Autodesk Inventor part; units mm, degrees
ref_plane "YZ Plane" through (0, 0, 0) normal (1, 0, 0) x (0, 1, 0)
ref_plane "XZ Plane" through (0, 0, 0) normal (0, 1, 0) x (-1, 0, 0)
ref_plane "XY Plane" through (0, 0, 0) normal (0, 0, 1) x (1, 0, 0)
sketch "Sketch1" plane through (0, 0, 0) normal (0, 0, 1) x (1, 0, 0)
  circle A0 centre (202.1451, 12.6471) radius 3.9688
  circle A1 centre (202.1451, -12.7529) radius 3.9688
  circle A2 centre (176.7451, 12.6471) radius 3.9688
  circle A3 centre (176.7451, -12.7529) radius 3.9688
  line L0 (211.6701, 22.1721) -> (167.2201, 22.1721)
  line L1 (167.2201, 22.1721) -> (167.2201, -22.2779)
  line L2 (167.2201, -22.2779) -> (211.6701, -22.2779)
  line L3 (211.6701, -22.2779) -> (211.6701, 22.1721)
  point P0 (0, 0)
  dimension "d0" = 9.525
  dimension "d1" = 9.525
  dimension "d2" = 44.45
  dimension "d3" = 44.45
extrude "Extrusion1" add sketch "Sketch1" along normal blind 38.1
sketch "Sketch2" plane through (0, 0, 38.1) normal (0, 0, 1) x (1, 0, 0)
  line L0 (211.6701, -22.2779) -> (211.6701, 22.1721)
  line L1 (167.2201, 22.1721) -> (167.2201, -22.2779)
  line L2 (211.6701, 22.1721) -> (167.2201, 22.1721)
  line L3 (167.2201, 22.1721) -> (167.2201, -22.2779)
  line L4 (167.2201, -22.2779) -> (211.6701, -22.2779)
  line L5 (211.6701, -22.2779) -> (211.6701, 22.1721)
  point P0 (0, 0)
extrude "Extrusion2" add sketch "Sketch2" along normal blind 165.1
sketch "Sketch3" plane through (167.2201, -22.2779, 0) normal (-1, 0, 0) x (0, 0, 1)
  point P0 (0, 22.2779)
sketch "Sketch4" plane through (211.6701, -22.2779, 0) normal (1, 0, 0) x (0, 0, -1)
  circle A0 centre (-127, 22.2779) radius 17.4625
  point P0 (0, 22.2779)
  dimension "d8" = 34.925
  dimension "d11" = 127
extrude "Extrusion3" cut sketch "Sketch4" against normal blind 7.1437
sketch "Sketch5" plane through (204.5263, 0, 127) normal (1, 0, 0) x (0, 0, -1)
  circle A0 centre (0, 0) radius 9.525
  point P0 (127, 0)
  dimension "d12" = 19.05
extrude "Extrusion4" cut sketch "Sketch5" against normal blind 50.8
sketch "Sketch6" plane through (167.2201, -22.2779, 0) normal (0, -1, 0) x (1, 0, 0)
  circle A0 centre (22.225, 171.45) radius 12.7
  line L0 (0, 203.2) -> (44.45, 203.2)
  point P0 (-167.2201, 0)
  dimension "d15" = 25.4
  dimension "d16" = 31.75
extrude "Extrusion5" cut sketch "Sketch6" against normal blind 50.8
sketch "Sketch7" plane through (167.2201, -22.2779, 0) normal (0, -1, 0) x (1, 0, 0)
  line L0 (44.45, 203.2) -> (0, 203.2)
  line L1 (23.8125, 203.2) -> (20.6375, 203.2)
  line L2 (20.6375, 203.2) -> (20.6375, 177.8)
  line L3 (20.6375, 177.8) -> (23.8125, 177.8)
  line L4 (23.8125, 177.8) -> (23.8125, 203.2)
  line L5 (44.45, 0) -> (44.45, 203.2)
  point P0 (-167.2201, 0)
  dimension "d19" = 3.175
  dimension "d20" = 20.6375
  dimension "d21" = 25.4
extrude "Extrusion6" cut sketch "Sketch7" against normal blind 50.8
sketch "Sketch8" plane through (211.6701, -22.2779, 0) normal (1, 0, 0) x (0, 0, -1)
  circle A0 centre (-193.675, 31.75) radius 6.35
  line L0 (-203.2, 0) -> (-203.2, 44.45)
  circle A1 centre (-193.675, 12.7) radius 6.35
  line L1 (0, 44.45) -> (-203.2, 44.45)
  line L2 (0, 0) -> (-203.2, 0)
  point P0 (0, 22.2779)
  dimension "d24" = 12.7
  dimension "d25" = 9.525
  dimension "d26" = 12.7
  dimension "d27" = 12.7
  dimension "d28" = 12.7
extrude "Extrusion7" cut sketch "Sketch8" against normal blind 7.9375
sketch "Sketch9" plane through (203.7326, 9.4721, 193.675) normal (1, 0, 0) x (0, 0, -1)
  circle A0 centre (0, 0) radius 6.35
  circle A1 centre (0, 0) radius 3.9688
  circle A2 centre (0, -19.05) radius 6.35
  circle A3 centre (0, -19.05) radius 3.9688
  point P0 (193.675, -9.4721)
  dimension "d31" = 7.9375
  dimension "d32" = 7.9375
extrude "Extrusion8" cut sketch "Sketch9" against normal blind 38.1 contours A1 | A3
properties part number "Corner Stand"
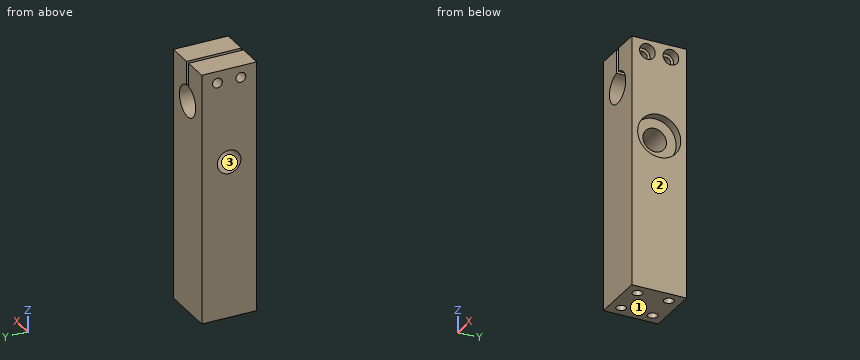
For this review, take the finished solid that the model builds, in its own axes (mm). Face numbers are marked on the shaded views. Coordinates: 2 decimals unless noted, no trailing zeros. Write each loop counter-clockwise with the first axis right and the second up, starting at its lowest first coordinate (ties: lowest second). Pieces come first, ordered by that corner, then holes. Notation, with made-up numbers: (66, 3.5) - (78, 3.5) arc R23 ccw to (78, 30.5) - close; hole circle Ø1 at (88.25, 67.5). An arc over 180 degrees is marked (long way). Answer in a Markdown table with one row per item. Add a question column.
Q1. For probe 1 along Z at (x, y) = (183.5, 6.5); probe 2 along Z at (x, y) = (208, -4); probe 3 along X at (y, z) = (-9.5, 131), list the stretches that pass through material, from the lowest coordinate up.
Q2. We need section D-D, the plane z = 18. State the section outline as (x, y) points, and give its area (3 significant figures).
Q3. Draft analysis for pull direction Z (two halves, no side actions). For the marked faces 1, 2 and 3, state which applies: +Z half, -Z half, draft (parallel to the pull), parting line (faces both ways), or undercut.
Q4. For P1, Ø6.5, axis at y = 9.47, z = 193.68, coming from the -X side; P2, Ø4, axis at x = 200.5, y = 12, coming from the -Z side; P3, Ø12.5, axis at y = -9.58, z = 193.68, coming from the +X side, all flat-tipped, find the tip position at first contact; note any pin that passes through.
Q5. We need section A-A, the plane z = 127. State the section outline as (x, y) points (1 decimal), and give its area (3 significant figures).
Q6. We need section C-C, the plane x = 184. State the section outline as (y, z) points (3 decimals), and give its area (3 significant figures).
Answer list:
| question | item | result |
|---|---|---|
| 1 | probe 1 | z = 0 to 120.04, 133.96 to 160.23, 182.67 to 191.04, 196.31 to 203.2 |
| 1 | probe 2 | z = 0 to 110, 144 to 190.64, 196.71 to 203.2 |
| 1 | probe 3 | x = 167.22 to 204.53 |
| 2 | outline | (167.22, -22.28) - (211.67, -22.28) - (211.67, 22.17) - (167.22, 22.17) - close; hole circle Ø7.94 at (176.75, -12.75); hole circle Ø7.94 at (176.75, 12.65); hole circle Ø7.94 at (202.15, -12.75); hole circle Ø7.94 at (202.15, 12.65) |
| 2 | area | 1,780 mm2 |
| 3 | face 1 | -Z half |
| 3 | face 2 | draft |
| 3 | face 3 | undercut |
| 4 | P1 | passes through |
| 4 | P2 | stops at z = 38.1 |
| 4 | P3 | stops at x = 203.73 |
| 5 | outline | (167.2, -22.3) - (211.7, -22.3) - (211.7, -17.5) - (204.5, -17.5) - (204.5, -9.5) - (167.2, -9.5) - close; (167.2, 9.5) - (204.5, 9.5) - (204.5, 17.5) - (211.7, 17.5) - (211.7, 22.2) - (167.2, 22.2) - close |
| 5 | area | 1,020 mm2 |
| 6 | outline | (-22.278, 0) - (22.172, 0) - (22.172, 159.977) - (-22.278, 159.977) - close; (-22.278, 182.923) - (22.172, 182.923) - (22.172, 203.2) - (-22.278, 203.2) - close; hole circle Ø7.938 at (-9.578, 193.675); hole circle Ø19.05 at (0, 127); hole circle Ø7.938 at (9.472, 193.675) |
| 6 | area | 7,630 mm2 |
